Part model, mm, in its own coordinate system. A direction names the side the tool comes from. Give positions to 0.01 mm unless a question says otherwise; leave off trailing zeros. Order: outer loops, then holes, each group sorted by start corner. A loop starts at its lowest first (then second) coordinate and runs counter-clockwise, first axis right, second up. Notation, with made-up numbers: M 30.25,-2.5 L 59.25,-2.5 A8 cw 59.25,4.5 Z; hole C 89,0.5 d5. An arc over 180 degrees is marked long. Return JSON: item names as keys, results as strings.
from build123d import *

# Parameters (mm, degrees)
PAD_DEPTH        = 15
HOLE_D           = 3.7
HOLE_CSINK_D     = 6.1
HOLE_CSINK_ANGLE = 90


with BuildPart() as part:
    # Sketch → Pad (new body)
    with BuildSketch(Plane.XY):
        with BuildLine():
            Line((0, 0), (-30, 0))
            Line((-30, 0), (-30, -15))
            Line((-30, -15), (0, -15))
            ThreePointArc((0, -15), (13.482659, -23.352651), (12.990381, -7.5))
            Line((27.990381, 18.480762), (12.990381, -7.5))
            Line((15, 25.980762), (27.990381, 18.480762))
            Line((0, 0), (15, 25.980762))
        make_face()
    extrude(amount=PAD_DEPTH)

    # Hole (through all)
    with Locations(Plane.XY.offset(15)):
        with Locations((8.982659, -15.558422)):
            CounterSinkHole(HOLE_D / 2, HOLE_CSINK_D / 2, counter_sink_angle=HOLE_CSINK_ANGLE)


solid = part.part
Q1. Band-saw the part on B-B (z = 8.25). Give the cut face in (x, y), then the cut area to 3 significant figures.
Established:
{"outline": "M -30,-15 L 0,-15 A9 ccw long 12.99,-7.5 L 27.99,18.48 L 15,25.98 L 0,0 L -30,0 Z; hole C 8.98,-15.56 d3.7", "area": "1,200 mm²"}
Q2. Two-plate mould, pull along X, no slides. Class faces 1 (the flat face through (-15, 0, 7)), 2 (the flat face through (21.404, 22.283, 7.395)), 3 (the cylindrical face through (10.35, -14.31, 6.8)): +X half, -X half, draft (parallel to the pull), parting line (faces both ways), or undercut.
Established:
{"face 1": "draft", "face 2": "+X half", "face 3": "undercut"}
Q3. Band-saw the part on C-C (y = 8.5). Give the cut face in (x, z), then the cut area to 3 significant figures.
Established:
{"outline": "M 4.91,0 L 22.23,0 L 22.23,15 L 4.91,15 Z", "area": "260 mm²"}
Q4. Band-saw the part on A-A (x = -5). Give the cut face in (y, z), then the cut area to 3 significant figures.
Established:
{"outline": "M -15,0 L 0,0 L 0,15 L -15,15 Z", "area": "225 mm²"}
Q5. Pin check, flat tips, straight feed: pin 1 (4 mm diameter, centred on x = -23, z = 3.5, fed in from -Y); pin 2 (7.5 mm diameter, centred on x = -11, z = 10, fed in from +Y); pin 3 (6 mm diameter, centred on x = 0, z = 12.5, fed in from -Y); pin 4 (3 mm diameter, centred on x = 8.98, y = -15.56, fed in from -Z). Stop position of each tip, or through.
Established:
{"pin 1": "stops at y = -15", "pin 2": "stops at y = 0", "pin 3": "stops at y = -22.28", "pin 4": "passes through"}
Q6. Probe line 1 along Y through (x, z) = (-3.5, 1.5); line 2 along Y through (x, z) = (25.5, 6.25); line 3 along X through (y, z) = (-17.5, 13.5). List the from-to ranges inside material, lowest first.
Established:
{"line 1": "y = -15 to 0", "line 2": "y = 14.17 to 19.92", "line 3": "x = 0.19 to 17.77"}
Q7. 3-axis set-ups, long thin cutter, end or side, ignore diameter. For faces 4 (the flat face through (-15, -15, 7)), 5 (the flat face through (20.595, 5.672, 7.395)), 6 (the flat face through (7.395, 12.809, 7.395)): which of +Z, -Z, +X, -X, +Y, -Y reach the whole face in a straight line?
Established:
{"face 4": "+Z, -Z, -X, -Y", "face 5": "+Z, -Z, +X", "face 6": "+Z, -Z, -X, +Y"}
